The model under review builds one solid part; all positions refer to its coordinate system, in mm. Give positions to 0.01 mm unless a question says otherwise; leave off trailing zeros. Order: outer loops, then holes, each group sorted by start corner. A loop starts at its lowest first (then second) coordinate and runs counter-clockwise, first axis right, second up.
```python
from build123d import *

# Parameters (mm, degrees)
SKETCH_1_R          = 12.5
EXTRUDE_1_DEPTH     = 358.6
CUT_EXTRUDE_START   = -30
SKETCH_2_W          = 8
SKETCH_2_H          = 8
CUT_EXTRUDE_1_DEPTH = 30
SKETCH_3_R          = 26
SKETCH_3_R_2        = 11.75
CUT_EXTRUDE_2_DEPTH = 1.7
CUT_EXTRUDE_START_2 = -128
SKETCH_4_W          = 8
SKETCH_4_H          = 8
CUT_EXTRUDE_3_DEPTH = 128
M10X1_252_D         = 8.8
M10X1_252_DEPTH     = 32.5
M10X1_252_TIP       = 2.643786724
M10X1_253_D         = 8.8
M10X1_253_DEPTH     = 32.5
M10X1_253_TIP       = 2.643786724


with BuildPart() as part:
    # Эскиз1 → Бобышка-Вытянуть1 (new body)
    with BuildSketch(Plane.XY):
        with Locations((0, -291.807573628)):
            Circle(SKETCH_1_R)
    extrude(amount=-EXTRUDE_1_DEPTH)

    # Эскиз2 → Вырез-Вытянуть1 (cut)
    with BuildSketch(Plane.XY.offset(CUT_EXTRUDE_START)):
        with Locations((-12.5, -291.807573628)):
            Rectangle(SKETCH_2_W, SKETCH_2_H)
    extrude(amount=CUT_EXTRUDE_1_DEPTH, mode=Mode.SUBTRACT)

    # Эскиз3 → Вырез-Вытянуть2 (cut)
    with BuildSketch(Plane(origin=(0, 0, -230.6), x_dir=(-1, 0, 0), z_dir=(0, 0, -1))):
        with Locations((0, -291.807573628)):
            Circle(SKETCH_3_R)
        with Locations((0, -291.807573628)):
            Circle(SKETCH_3_R_2, mode=Mode.SUBTRACT)
    extrude(amount=-CUT_EXTRUDE_2_DEPTH, mode=Mode.SUBTRACT)

    # Эскиз4 → Вырез-Вытянуть3 (cut)
    with BuildSketch(Plane(origin=(0, 0, -358.6), x_dir=(-1, 0, 0), z_dir=(0, 0, -1)).offset(CUT_EXTRUDE_START_2)):
        with Locations((12.5, -291.807573628)):
            Rectangle(SKETCH_4_W, SKETCH_4_H)
    extrude(amount=CUT_EXTRUDE_3_DEPTH, mode=Mode.SUBTRACT)

    # Сверление под метчик M10x1.252
    with Locations(Plane.XY):
        with Locations((0, -291.807573628)):
            Hole(M10X1_252_D / 2, depth=M10X1_252_DEPTH)
            with Locations((0, 0, -(M10X1_252_DEPTH + M10X1_252_TIP / 2))):  # 118° drill point
                Cone(0, M10X1_252_D / 2, M10X1_252_TIP, mode=Mode.SUBTRACT)

    # Сверление под метчик M10x1.253
    with Locations(Plane(origin=(0, 0, -358.6), x_dir=(-1, 0, 0), z_dir=(0, 0, -1))):
        with Locations((0, -291.807573628)):
            Hole(M10X1_253_D / 2, depth=M10X1_253_DEPTH)
            with Locations((0, 0, -(M10X1_253_DEPTH + M10X1_253_TIP / 2))):  # 118° drill point
                Cone(0, M10X1_253_D / 2, M10X1_253_TIP, mode=Mode.SUBTRACT)


solid = part.part
```
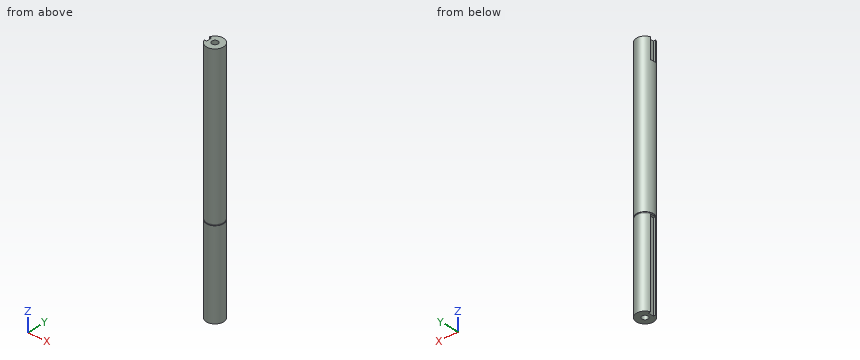
Item 1: Take a section at B-B (x = 8.5). Give the boundary of the cut face in (y, z), and give its area (3 significant figures).
Values found:
outline: (-300.97, -358.6) - (-282.64, -358.6) - (-282.64, -230.6) - (-283.7, -230.6) - (-283.7, -228.9) - (-282.64, -228.9) - (-282.64, 0) - (-300.97, 0) - (-300.97, -228.9) - (-299.92, -228.9) - (-299.92, -230.6) - (-300.97, -230.6) - close
area: 6,570 mm2
Item 2: Clearance check with flat-ended pins moving along their axes: pin 1 Ø5 at (x, z) = (10, -44) entering from +Y; pin 2 Ø9 at (y, z) = (-293, -8.5) entering from -X; pin 3 Ø6.5 at (y, z) = (-292, -299.5) entering from -X; pin 4 Ø4 at (x, y) = (-4.5, -298.5) entering from +Z. State where each tip first meets the part, or that it passes through.
Values found:
pin 1: stops at y = -281.81
pin 2: stops at x = -11.84
pin 3: stops at x = -8.5
pin 4: stops at z = 0
Item 3: For line 1 (Y direction, x = 0, z = -346); line 2 (Z direction, x = 10.75, y = -286); line 3 (Y direction, x = 0, z = -301.5), list the stretches that pass through material, from the lowest coordinate up.
Values found:
line 1: y = -304.31 to -296.21, -287.41 to -279.31
line 2: z = -358.6 to -230.6, -228.9 to 0
line 3: y = -304.31 to -279.31
Item 4: Take a section at A-A (y = -300.5). Give the boundary of the cut face in (x, z), and give its area (3 significant figures).
Values found:
outline: (-8.98, -358.6) - (8.98, -358.6) - (8.98, -230.6) - (7.91, -230.6) - (7.91, -228.9) - (8.98, -228.9) - (8.98, 0) - (-8.98, 0) - (-8.98, -228.9) - (-7.91, -228.9) - (-7.91, -230.6) - (-8.98, -230.6) - close
area: 6,440 mm2
Item 5: Take a section at C-C (z = -213). Give the boundary of the cut face in (x, y), and give its area (3 significant figures).
Values found:
outline: circle Ø25 at (0, -291.81)
area: 491 mm2
